Here's how the part is built. I have some questions about the finished solid (model axes, mm). A direction names the side the tool comes from. Round coordinates to 2 decimals unless told otherwise and drop trailing zeros. Order: outer loops, then holes, each group sorted by start corner. A loop starts at its lowest first (then second) coordinate and runs counter-clockwise, first axis right, second up. Notation, with made-up numbers: (22, -30) - (62, -30) arc R29 cw to (62, 2) - close; hole circle Ø11 at (78, 27.5). An arc over 180 degrees is marked (long way). Answer as a JSON object with one key per item and string values.
```python
from build123d import *

# Parameters (mm, degrees)
SKETCH1_W           = 25.4
SKETCH1_H           = 25.4
BOSS_EXTRUDE2_DEPTH = 584.2
SKETCH2_W           = 20.302766191
SKETCH2_H           = 19.05
CUT_EXTRUDE1_DEPTH  = 586.303305988
CUT_EXTRUDE2_DEPTH  = 586.303305988
SKETCH6_R           = 3.175
CUT_EXTRUDE5_DEPTH  = 586.303306096
SKETCH4_W           = 6.35
SKETCH4_H           = 41.278824243
CUT_EXTRUDE6_DEPTH  = 586.303306096


with BuildPart() as part:
    # Sketch1 → Boss-Extrude2 (new body)
    with BuildSketch(Plane.XY):
        with Locations((12.7, 12.7)):
            Rectangle(SKETCH1_W, SKETCH1_H)
    extrude(amount=BOSS_EXTRUDE2_DEPTH)

    # Sketch2 → Cut-Extrude1 (cut, through all)
    with BuildSketch(Plane(origin=(0, 0, 0), x_dir=(-1, 0, 0), z_dir=(0, 0, -1))):
        with Locations((-13.326383096, 12.7)):
            Rectangle(SKETCH2_W, SKETCH2_H)
    extrude(amount=-CUT_EXTRUDE1_DEPTH, mode=Mode.SUBTRACT)

    # Sketch3 → Cut-Extrude2 (cut, through all)
    with BuildSketch(Plane(origin=(0, 25.4, 0), x_dir=(1, 0, 0), z_dir=(0, 1, 0))):
        with BuildLine():
            add(Edge.make_bspline(
                [(12.7, 0), (0, 0), (0, -30.465860076)],
                knots=[6.283185307, 6.283185307, 6.283185307, 7.853981634, 7.853981634, 7.853981634], degree=2, weights=[1, 0.707106781, 1]))
            Line((12.7, 0), (0, 0))
            Line((0, 0), (0, -30.465860076))
        make_face()
        with BuildLine():
            Line((25.4, 0), (12.7, 0))
            add(Edge.make_bspline(
                [(25.4, -30.465860076), (25.4, 0), (12.7, 0)],
                knots=[4.71238898, 4.71238898, 4.71238898, 6.283185307, 6.283185307, 6.283185307], degree=2, weights=[1, 0.707106781, 1]))
            Line((25.4, -30.465860076), (25.4, 0))
        make_face()
    extrude(amount=-CUT_EXTRUDE2_DEPTH, mode=Mode.SUBTRACT)

    # Sketch6 → Cut-Extrude5 (cut, through all)
    with BuildSketch(Plane(origin=(0, 25.4, 0), x_dir=(1, 0, 0), z_dir=(0, 1, 0))):
        with Locations(Location((12.7, -12.7, 0), (0, 0, 270))):
            Circle(SKETCH6_R)
    extrude(amount=-CUT_EXTRUDE5_DEPTH, mode=Mode.SUBTRACT)

    # Sketch4 → Cut-Extrude6 (cut, through all)
    with BuildSketch(Plane(origin=(0, 25.4, 0), x_dir=(1, 0, 0), z_dir=(0, 1, 0))):
        with Locations((12.7, -258.760587879)):
            Rectangle(SKETCH4_W, SKETCH4_H)
    extrude(amount=-CUT_EXTRUDE6_DEPTH, mode=Mode.SUBTRACT)


solid = part.part
```
1. If I drill on L1, parallel to Y at x = 10, z = 423 (3 decimals); L2, parallel to X at y = 8.25, z = 238 (3 decimals); L3, parallel to Z at x = 14.5, y = 2, over which ranges is the centre line in solid material (lowest first)? Write a range as [from, to].
Responses:
{"L1": "[0, 3.175], [22.225, 25.4]", "L2": "[0, 3.175], [23.478, 25.4]", "L3": "[0.31, 10.08], [15.32, 238.12], [279.4, 584.2]"}
2. Imagine slicing it at A-A (z = 261). List the corners of the cut face in (x, y) for me (3 decimals).
Responses:
{"outline": "(0, 0) - (9.525, 0) - (9.525, 3.175) - (3.175, 3.175) - (3.175, 22.225) - (9.525, 22.225) - (9.525, 25.4) - (0, 25.4) - close; (15.875, 0) - (25.4, 0) - (25.4, 25.4) - (15.875, 25.4) - (15.875, 22.225) - (23.478, 22.225) - (23.478, 3.175) - (15.875, 3.175) - close"}
3. For faces 1 (the face through (23.478, 13, 295)), 2 (the face through (0, 13, 303)), which set-ups out of +Z, -Z, +X, -X, +Y, -Y let a thin tool reach every point of the face, with its end or its side?
Responses:
{"face 1": "+Z, -Z", "face 2": "+Z, -Z, -X, +Y, -Y"}
4. For P1, Ø6, axis at y = 9, z = 386.5, coming from the -X side; P2, Ø2.5, axis at x = 11, y = 24.5, coming from the -Z side; P3, Ø8, axis at x = 11.5, y = 14.5, coming from the -Z side, each with a flat end and sliding along its axis, tell me the tip position at first contact or that it passes through.
Responses:
{"P1": "x = 0", "P2": "z = 0.02", "P3": "through"}
5. Thinking about a two-plate mould opening in X: for faces 3 (the face through (13, 25.4, 288)), 4 (the face through (13, 22.225, 288)), 5 (the face through (25.4, 13, 303)), which applies, pulls with the +X half, pulls with the -X half, needs draft (parallel to the pull), parting line crosses it, or undercut?
Responses:
{"face 3": "needs draft", "face 4": "undercut", "face 5": "pulls with the +X half"}
